```python
from build123d import *

# Parameters (mm, degrees)
SKETCH1_R           = 2.5
BOSS_EXTRUDE1_DEPTH = 5
SKETCH2_R           = 10
BOSS_EXTRUDE2_DEPTH = 40
CUT_EXTRUDE1_REACH  = 53.609
SKETCH3_R           = 8


with BuildPart() as part:
    # Sketch1 → Boss-Extrude1 (new body)
    with BuildSketch(Plane.XY):
        with BuildLine():
            Line((-19.339079606, -11.5), (19.339079606, -11.5))
            ThreePointArc((19.339079606, -11.5), (22.5, 0), (19.339079606, 11.5))
            Line((19.339079606, 11.5), (-19.339079606, 11.5))
            ThreePointArc((-19.339079606, 11.5), (-22.5, 0), (-19.339079606, -11.5))
        make_face()
        with Locations((-16.5, 0)):
            Circle(SKETCH1_R, mode=Mode.SUBTRACT)
        with Locations((16.5, 0)):
            Circle(SKETCH1_R, mode=Mode.SUBTRACT)
    extrude(amount=BOSS_EXTRUDE1_DEPTH)

    # Sketch2 → Boss-Extrude2 (add)
    with BuildSketch(Plane(origin=(0, 0, 0), x_dir=(-1, 0, 0), z_dir=(0, 0, -1))):
        with Locations(Location((0, 0, 0), (0, 0, 180))):
            Circle(SKETCH2_R)
    extrude(amount=BOSS_EXTRUDE2_DEPTH)

    # Sketch3 → Cut-Extrude1 (cut, up to next)
    with BuildSketch(Plane.XY.offset(5), mode=Mode.PRIVATE) as cut_extrude1_sk1:
        Circle(SKETCH3_R)
    cut_extrude1_tool1 = extrude(cut_extrude1_sk1.sketch, amount=-CUT_EXTRUDE1_REACH, mode=Mode.PRIVATE) & part.part
    add(cut_extrude1_tool1.solids().sort_by_distance((0, 0, 5))[0], mode=Mode.SUBTRACT)


solid = part.part
```
Design review of the part built by this model. Coordinates are the model's own, in mm. Give positions to 0.01 mm unless a question says otherwise; leave off trailing zeros. Order: outer loops, then holes, each group sorted by start corner. A loop starts at its lowest first (then second) coordinate and runs counter-clockwise, first axis right, second up. Notation, with made-up numbers: M 51,65 L 73,65 A17 cw 73,92 Z; hole C -9.75,-14 d4. An arc over 180 degrees is marked long. One line per question, with ' | ' between items. Start each with the question number.
Q1. For L1, parallel to Y at x = -16.5, z = 3.25; L2, parallel to Y at x = 16, z = 1; L3, parallel to Z at x = 8, y = 7.75, list the stretches that pass through material, from the lowest coordinate up. Write a range as [from, to].
Q2. The part is to be moulded in two halves that separate along X. For faces 1 (the face through (0, -11.5, 2)), 2 (the face through (-19, 0, 2)), 3 (the face through (14, 0, 2)), 4 (the face through (-10, 0, -20)), say which applies: +X half, -X half, draft (parallel to the pull), parting line (faces both ways), or undercut.
Q3. We need section D-D (y = -5). Write out the cut boundary in (x, z) (3 decimals).
Q4. We need section B-B (z = 1). Write out the cut boundary in (x, y).
Q5. For pin 1 Ø6.5 at (x, y) = (-16.5, 0) entering from -Z; pin 2 Ø4 at (y, z) = (3.5, -31) entering from +X; pin 3 Ø1 at (y, z) = (-5, -9.5) entering from -X; pin 4 Ø3 at (x, y) = (4.5, 5) entering from +Z, all flat-tipped, find the tip position at first contact; note any pin that passes through.
Q6. We need section C-C (y = 1.5). Write out the cut boundary in (x, z).
Q7. We need section A-A (x = -16.5). Write out the cut boundary in (y, z).
Returned:
1) L1: [-11.5, -2.5], [2.5, 11.5] | L2: [-11.5, -2.45], [2.45, 11.5] | L3: [0, 5]
2) face 1: draft | face 2: undercut | face 3: undercut | face 4: parting line
3) outline: M -21.937,0 L -8.66,0 L -8.66,-40 L -6.245,-40 L -6.245,5 L -21.937,5 Z; M 6.245,-40 L 8.66,-40 L 8.66,0 L 21.937,0 L 21.937,5 L 6.245,5 Z
4) outline: M -19.34,-11.5 L 19.34,-11.5 A22.5 ccw 19.34,11.5 L -19.34,11.5 A22.5 ccw Z; hole C -16.5,0 d5; hole C 0,0 d16; hole C 16.5,0 d5
5) pin 1: z = 0 | pin 2: x = 9.89 | pin 3: x = -8.93 | pin 4: z = 5
6) outline: M -22.45,0 L -18.5,0 L -18.5,5 L -22.45,5 Z; M -14.5,0 L -9.89,0 L -9.89,-40 L -7.86,-40 L -7.86,5 L -14.5,5 Z; M 7.86,-40 L 9.89,-40 L 9.89,0 L 14.5,0 L 14.5,5 L 7.86,5 Z; M 18.5,0 L 22.45,0 L 22.45,5 L 18.5,5 Z
7) outline: M -11.5,0 L -2.5,0 L -2.5,5 L -11.5,5 Z; M 2.5,0 L 11.5,0 L 11.5,5 L 2.5,5 Z
